```python
from build123d import *

# Parameters (mm, degrees)
EXTRUDE_1_DEPTH     = 20
SKETCH_2_W          = 25
SKETCH_2_H          = 4
CUT_EXTRUDE_1_DEPTH = 20
CUT_EXTRUDE_START   = -3
SKETCH_3_W          = 10
SKETCH_3_H          = 16
CUT_EXTRUDE_2_DEPTH = 30
SKETCH_4_R          = 1.330699037
CUT_EXTRUDE_3_DEPTH = 3
FILLET_2_R          = 5
FILLET_3_R          = 5


with BuildPart() as part:
    # Эскиз1 → Бобышка-Вытянуть1 (new body)
    with BuildSketch(Plane(origin=(0, 0, 0), x_dir=(1, 0, 0), z_dir=(0, 1, 0))):
        Polygon((0, 0), (0, 30), (40, 15), align=None)
    extrude(amount=EXTRUDE_1_DEPTH)

    # Эскиз2 → Вырез-Вытянуть1 (cut)
    with BuildSketch(Plane(origin=(0, 20, 0), x_dir=(1, 0, 0), z_dir=(0, 1, 0))):
        with Locations((12.5, 15)):
            Rectangle(SKETCH_2_W, SKETCH_2_H)
    extrude(amount=-CUT_EXTRUDE_1_DEPTH, mode=Mode.SUBTRACT)

    # Эскиз3 → Вырез-Вытянуть2 (cut)
    with BuildSketch(Plane.ZY.offset(CUT_EXTRUDE_START)):
        with Locations((-25, 10)):
            Rectangle(SKETCH_3_W, SKETCH_3_H)
        with Locations((-5, 10)):
            Rectangle(SKETCH_3_W, SKETCH_3_H)
    extrude(amount=-CUT_EXTRUDE_2_DEPTH, mode=Mode.SUBTRACT)

    # Эскиз4 → Вырез-Вытянуть3 (cut)
    with BuildSketch(Plane.ZY):
        with Locations((-25, 10)):
            Circle(SKETCH_4_R)
        with Locations((-5, 10)):
            Circle(SKETCH_4_R)
    extrude(amount=-CUT_EXTRUDE_3_DEPTH, mode=Mode.SUBTRACT)

    # Скругление2
    fillet_2_edges = [part.edges().sort_by_distance(p)[0] for p in [
        (40, 10, -15),
    ]]
    fillet(fillet_2_edges, radius=FILLET_2_R)

    # Скругление3
    fillet_3_edges = [part.edges().sort_by_distance(p)[0] for p in [
        (14.833333333, 18, -20),
        (14.833333333, 2, -20),
        (3, 2, -24.4375),
        (3, 18, -24.4375),
        (14.833333333, 2, -10),
        (14.833333333, 18, -10),
        (3, 18, -5.5625),
        (3, 2, -5.5625),
    ]]
    fillet(fillet_3_edges, radius=FILLET_3_R)


solid = part.part
```
Work out the finished part from the listing and answer in its coordinate system (mm). A direction names the side the tool comes from. Give positions to 0.01 mm unless a question says otherwise; leave off trailing zeros. Loops run counter-clockwise (first coordinate to the right, second up) from the corner with the lowest first, then second, coordinate; pieces in that order, holes last. Notation, with made-up numbers: (-30, 82.5) - (10, 82.5) arc R15 cw to (10, 99.5) - close; hole circle Ø8 at (-32, 51). An arc over 180 degrees is marked (long way). Use CSV: the item, a comma, the result in double quotes. Start each with the question number.
(1) Find section D-D, the plane y = 7.75. Determine the outline of the cut face in (x, z) (3 decimals), plus the area to 3 significant figures.
(2) Find section B-B, the plane y = 10. Determine the outline of the cut face in (x, z) (3 decimals).
(3) Find section A-A, the plane x = 2. Determine the outline of the cut face in (y, z), plus the area to 3 significant figures.
(4) Determine the mould class of faces 6 (the face through (15, 16, -9)), 7 (the face through (0, 10, -8)), 8 (the face through (1.479, 8.819, -4.386)) for opening direction Z: released by +Z, released by -Z, zero draft, split by the parting line, or undercut.
(5) A tool of negligible diameter and unlimited length cuts with its end or side. For faces 1 (the face through (15, 16, -21)), 2 (the face through (12, 0, -12)), 3 (the face through (12, 10, -17)), 4 (the face through (4, 4, -6)), 5 (the face through (12, 20, -12)), from which of +Z, -Z, +X, -X, +Y, -Y can it reach the whole face along a straight path? Write none if from no direction.
(6) Find section C-C, the plane z = -4.5. Determine the outline of the cut face in (x, y).
(7) Each of these flat-tipped pins is pushed along its axis until it touches: pin 1 (3 mm diameter, centred on y = 9, z = -25, fed in from +X); pin 2 (6 mm diameter, centred on x = 11, y = 8.5, fed in from +Z); pin 3 (3 mm diameter, centred on x = 10.5, y = 9.5, fed in from +Z). Where does it stop, or does it pass through?
(8) Find the intervals of material crossed by L1, parallel to Y at x = 1.3, z = -5; L2, parallel to Y at x = 9.5, z = -25.5; L3, parallel to X at y = 7.75, z = -6, in increasing order.
Results found:
1,outline,"(0, -30) - (3, -28.875) - (3, -20) - (26.667, -20) - (27.516, -19.682) arc R5 ccw to (27.516, -10.318) - (26.667, -10) - (3, -10) - (3, -1.125) - (0, 0) - (0, -13) - (25, -13) - (25, -17) - (0, -17) - close"
1,area,"254 mm^2"
2,outline,"(0, -30) - (3, -28.875) - (3, -26.331) - (0, -26.331) - close; (0, -23.669) - (3, -23.669) - (3, -20) - (26.667, -20) - (27.516, -19.682) arc R5 ccw to (27.516, -10.318) - (26.667, -10) - (3, -10) - (3, -6.331) - (0, -6.331) - (0, -13) - (25, -13) - (25, -17) - (0, -17) - close; (0, -3.669) - (3, -3.669) - (3, -1.125) - (0, 0) - close"
3,outline,"(0, -29.25) - (20, -29.25) - (20, -17) - (0, -17) - close; (0, -13) - (20, -13) - (20, -0.75) - (0, -0.75) - close; hole circle Ø2.66 at (10, -25); hole circle Ø2.66 at (10, -5)"
3,area,"479 mm^2"
4,face 6,"released by +Z"
4,face 7,"zero draft"
4,face 8,"undercut"
5,face 1,"-Z, +X"
5,face 2,"+Z, -Z, +X, -X, -Y"
5,face 3,"-X, +Y, -Y"
5,face 4,"+Z, +X"
5,face 5,"+Z, -Z, +X, -X, +Y"
6,outline,"(0, 0) - (12, 0) - (12, 2) - (8, 2) arc R5 cw to (3, 7) - (3, 8.77) - (0, 8.77) - close; (0, 11.23) - (3, 11.23) - (3, 13) arc R5 cw to (8, 18) - (12, 18) - (12, 20) - (0, 20) - close"
7,pin 1,"x = 3"
7,pin 2,"z = -9.77"
7,pin 3,"z = -10"
8,L1,"0 to 8.67, 11.33 to 20"
8,L2,"0 to 2, 18 to 20"
8,L3,"0 to 3"
